from build123d import *


with BuildPart() as f1:
    # F0 (on Front) → F1 (revolve)
    with BuildSketch(Plane.XZ):
        with BuildLine():
            Line((-5.969, 9.596622), (-5.969, 24.892))
            Line((-5.969, 24.892), (-8.412302, 26.384082))
            Line((-8.412302, 26.384082), (-13.589, 26.384082))
            Line((-13.589, 26.384082), (-13.589, 12.002977))
            ThreePointArc((-13.589, 12.002977), (-15.448872, 7.512849), (-19.939, 5.652977))
            Line((-19.939, 5.652977), (-23.33023, 5.652977))
            Line((-23.33023, 5.652977), (-26.593978, 0))
            Line((-26.593978, 0), (0, 0))
            Line((0, 0), (0, 8.731734))
            Line((0, 8.731734), (-5.104112, 8.731734))
            ThreePointArc((-5.104112, 8.731734), (-5.71568, 8.985054), (-5.969, 9.596622))
        make_face()
    revolve(axis=Axis((0, 0, 12.446), (0, 0, 1)))


solid = f1.part
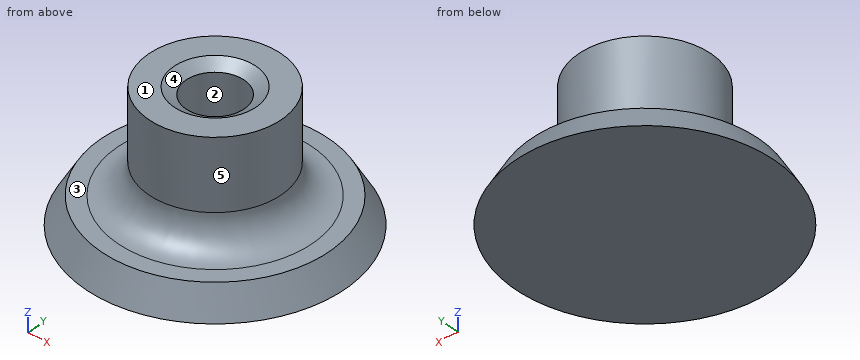
Geometry: final body of the model. Coordinates: model frame, mm. Face numbers are marked on the shaded views. A direction names the side the tool comes from. Give positions to 0.01 mm unless a question says otherwise; leave off trailing zeros. Write each loop counter-clockwise with the first axis right and the second up, starting at its lowest first coordinate (ties: lowest second). Pieces come first, ordered by that corner, then holes. Notation, with made-up numbers: (9, -35.75) - (57, -35.75) arc R16 ccw to (57, -20.75) - close; hole circle Ø1 at (14.5, 89). An arc over 180 degrees is marked (long way). Return JSON: item names as keys, results as strings. Group by question number.
1) Section C-C on z = 21.75. Return the cut outline in (x, y), plus the area to 3 significant figures.
2) Mould query, pull axis Y, two halves, no side actions, for the marked faces 3, 4 and 5. Classes: released by +Y, released by -Y, zero draft, split by the parting line, or undercut.
3) Line query: line 1 (X direction, y = 0, z = 18); line 2 (Z direction, x = 6.5, y = 22). Output: solid intervals per line, ascending.
4) Section A-A on x = 0. Return the cut outline in (y, z), plus the area to 3 significant figures.
5) Set-up query: the marked faces 1 and 2. Return all of +Z, -Z, +X, -X, +Y, -Y with unobstructed straight access to the full face (end or side cutting, diameter ignored); none if empty.
6) First-contact query: P1, Ø2, axis at y = -12, z = 11.5, coming from the -X side; P2, Ø5, axis at x = -1.5, z = 4.5, coming from the -Y side; P3, Ø3, axis at x = 12, z = 22, coming from the -Y side. Flat tips, straight axial feed; report the tip coordinate or a pass-through.
Filled in:
{
 "1": {"outline": "circle Ø27.18 at (0, 0); hole circle Ø11.94 at (0, 0)", "area": "468 mm^2"},
 "2": {"face 3": "zero draft", "face 4": "undercut", "face 5": "split by the parting line"},
 "3": {"line 1": "x = -13.59 to -5.97, 5.97 to 13.59", "line 2": "z = 0 to 5.65"},
 "4": {"outline": "(-26.59, 0) - (26.59, 0) - (23.33, 5.65) - (19.94, 5.65) arc R6.35 cw to (13.59, 12) - (13.59, 26.38) - (8.41, 26.38) - (5.97, 24.89) - (5.97, 9.6) arc R0.86 cw to (5.1, 8.73) - (-5.1, 8.73) arc R0.86 cw to (-5.97, 9.6) - (-5.97, 24.89) - (-8.41, 26.38) - (-13.59, 26.38) - (-13.59, 12) arc R6.35 cw to (-19.94, 5.65) - (-23.33, 5.65) - close", "area": "649 mm^2"},
 "5": {"face 1": "+Z, +X, -X, +Y, -Y", "face 2": "+Z"},
 "6": {"P1": "stops at x = -8.02", "P2": "stops at y = -25.4", "P3": "stops at y = -8.63"}
}
